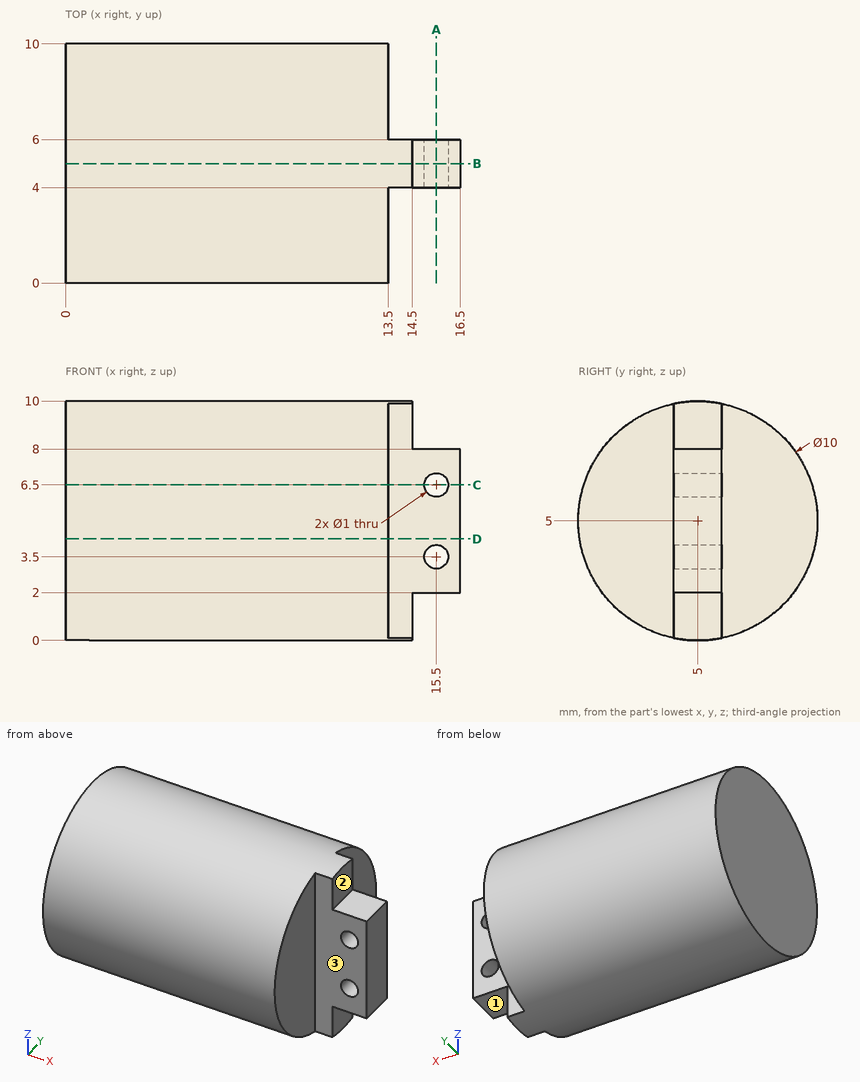
The figure shows three views and two pictorial views of one solid part (mm, origin at its lowest corner). Answer the questions. A direction names the side the tool comes from. Coordinates: 2 decimals unless noted, no trailing zeros. Write each loop counter-clockwise with the first axis right and the second up, starting at its lowest first coordinate (ties: lowest second). Pieces come first, ordered by that corner, then holes. Notation, with made-up numbers: (39.5, 52) -> (55.5, 52) arc R14 ccw to (55.5, 75) -> close; hole circle Ø5 at (54, -22). An arc over 180 degrees is marked (long way). Return JSON: item names as keys, results as strings.
(1) The part is cut by section C-C on z = 6.5. Give the vertices of the cut face in (x, y).
Answers below:
{"outline": "(0, 0.23) -> (13.5, 0.23) -> (13.5, 4) -> (15, 4) -> (15, 6) -> (13.5, 6) -> (13.5, 9.77) -> (0, 9.77) -> close; (16, 4) -> (16.5, 4) -> (16.5, 6) -> (16, 6) -> close"}
(2) The part is cut by section B-B on y = 5. Give the vertices of the cut face in (x, z), then the cut area to 3 significant figures.
Answers below:
{"outline": "(0, 0) -> (14.5, 0) -> (14.5, 2) -> (16.5, 2) -> (16.5, 8) -> (14.5, 8) -> (14.5, 10) -> (0, 10) -> close; hole circle Ø1 at (15.5, 3.5); hole circle Ø1 at (15.5, 6.5)", "area": "155 mm^2"}
(3) Which of the six approach directions +Z, -Z, +X, -X, +Y, -Y give full straight-line access (tool end or side, diameter ignored) to the marked faces 1, 2 and 3?
Answers below:
{"face 1": "-Z, +X, +Y, -Y", "face 2": "+Z, +X, +Y, -Y", "face 3": "+Z, -Z, +X, -Y"}
(4) Each of these flat-tipped pins is pushed along its axis until it touches: P1, Ø1, axis at x = 14.5, z = 7, coming from the +Y side; P2, Ø1, axis at y = 5, z = 9.5, coming from the +X side; P3, Ø1.6, axis at x = 15.5, y = 5.5, coming from the +Z side. Where does it stop, or does it pass through?
Answers below:
{"P1": "y = 6", "P2": "x = 14.5", "P3": "z = 8"}
(5) The part is cut by section A-A on x = 15.5. Give the vertices of the cut face in (y, z).
Answers below:
{"outline": "(4, 2) -> (6, 2) -> (6, 3) -> (4, 3) -> close; (4, 4) -> (6, 4) -> (6, 6) -> (4, 6) -> close; (4, 7) -> (6, 7) -> (6, 8) -> (4, 8) -> close"}
(6) Consider line 1 along Z through (x, y) = (15.5, 4.75); line 2 along X through (y, z) = (5.1, 6.5); line 3 along X through (y, z) = (2.75, 3.75). Determine where each line is inside the solid, lowest interval first. Write a range as from..to.
Answers below:
{"line 1": "2..3, 4..6, 7..8", "line 2": "0..15, 16..16.5", "line 3": "0..13.5"}
(7) The part is cut by section D-D on z = 4.25. Give the vertices of the cut face in (x, y).
Answers below:
{"outline": "(0, 0.06) -> (13.5, 0.06) -> (13.5, 4) -> (16.5, 4) -> (16.5, 6) -> (13.5, 6) -> (13.5, 9.94) -> (0, 9.94) -> close"}
